```python
from build123d import *

# Parameters (mm, degrees)
F1_DEPTH = 270
F2_T     = -7
F3_R     = 14.5182596714
F4_DEPTH = 25


with BuildPart() as f1:
    # F0 (on Top) → F1 (new body)
    with BuildSketch(Plane.XY):
        Polygon((47.4160599989, -68.5225782833), (80.3682735811, -22.0128844547), (75.7152787608, 34.7968826563), (35.6342635267, 75.3248016481), (-21.1204196422, 80.6074088069), (-67.9926237332, 48.1729135333), (-83.0503235256, -6.8022233647), (-59.2478539389, -58.5945243522), (-7.7226550276, -82.9697961896), align=None)
    extrude(amount=F1_DEPTH)

    # F2
    f2_openings = [f1.faces().sort_by_distance(p)[0] for p in [
        (0, 0, 270),
    ]]
    offset(amount=F2_T, openings=f2_openings)

    # F3 (on face) → F4 (cut)
    with BuildSketch(Plane(origin=(-33.4852544832, -70.7821602709, 0), x_dir=(0.9039508581, -0.427636348, 0), z_dir=(-0.427636348, -0.9039508581, 0))):
        with Locations((-6.3656242564, 136.8046998978)):
            Circle(F3_R)
    extrude(amount=-F4_DEPTH, mode=Mode.SUBTRACT)


solid = f1.part
```
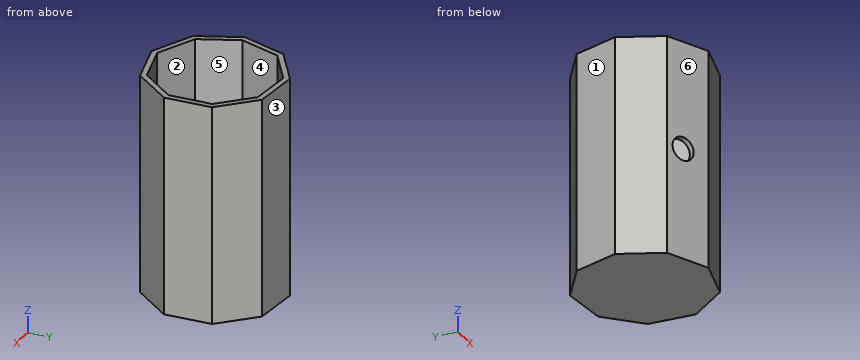
Verification items for the finished model (mm, model axes). Face numbers are marked on the shaded views. A direction names the side the tool comes from. Coordinates: 2 decimals unless noted, no trailing zeros. Write each loop counter-clockwise with the first axis right and the second up, starting at its lowest first coordinate (ties: lowest second). Pieces come first, ordered by that corner, then holes. Notation, with made-up numbers: (48.5, -24.5) - (70.5, -24.5) arc R18 cw to (70.5, -3.5) - close; hole circle Ø8 at (32.25, 62). An arc over 180 degrees is marked (long way). Write item = value, one per line.
Q1. Cross-section at C-C (y = 1). Enter the section's corners in (x, z).
Answer:
outline = (-80.91, 0) - (78.48, 0) - (78.48, 270) - (71.46, 270) - (71.46, 7) - (-73.66, 7) - (-73.66, 270) - (-80.91, 270) - close
Q2. Mould release check, pull along X, two halves, no side actions. Record for the marked faces 3, 4, 5 and 6: released by +X, released by -X, zero draft, split by the parting line, or undercut.
Answer:
face_3 = released by +X
face_4 = undercut
face_5 = undercut
face_6 = released by -X
Q3. Cross-section at A-A (z = 211.5). Enter the section's corners in (x, y), plus the area to 3 significant figures.
Answer:
outline = (-83.05, -6.8) - (-59.25, -58.59) - (-7.72, -82.97) - (47.42, -68.52) - (80.37, -22.01) - (75.72, 34.8) - (35.63, 75.32) - (-21.12, 80.61) - (-67.99, 48.17) - close; hole (-75.63, -6.19) - (-53.95, -53.36) - (-7.03, -75.55) - (43.18, -62.4) - (73.18, -20.05) - (68.95, 31.69) - (32.45, 68.59) - (-19.23, 73.4) - (-61.91, 43.87) - close
area = 3,430 mm²
Q4. Go/stop test with flat-tipped pins: pin 1 Ø1 at (x, y) = (36.5, 4.5) entering from +Z; pin 2 Ø10 at (x, z) = (1, 221.5) entering from -Y; pin 3 Ø5 at (y, z) = (61.5, 79) entering from -X. Record where each tip stops, or that it passes through.
Answer:
pin_1 = 7
pin_2 = -81.99
pin_3 = -52.35
Q5. Cross-section at B-B (x = -1.5). Enter the section's corners in (y, z).
Answer:
outline = (-81.34, 0) - (78.78, 0) - (78.78, 270) - (71.75, 270) - (71.75, 7) - (-74.1, 7) - (-74.1, 270) - (-81.34, 270) - close
Q6. Material ranges on L1, parallel to Z at x = -3.5, y = 53; L2, parallel to Y at x = 48, z = 134.5; L3, parallel to X at y = 22.5, z = 14.5, recorded low to high. Write a range as from..to.
Answer:
L1 = 0..7
L2 = -67.7..-55.59, 52.87..62.82
L3 = -75.02..-67.77, 69.7..76.72
Q7. Access from +Z, -Z, +X, -X, +Y, -Y to the whole of each face (thin tool, end or side, straight path). Record for the marked faces 1 and 2.
Answer:
face_1 = +Z, -Z, -X, +Y
face_2 = +Z
